```python
from build123d import *

# Parameters (mm, degrees)
F1_DEPTH  = 15
F2_DEPTH  = 15
F3_W      = 7.4589547733
F3_H      = 5.06
F4_DEPTH  = 25
F5_W      = 8.8782840291
F5_H      = 5.06
F6_DEPTH  = 25
F7_W      = 4.8981418308
F7_H      = 5.06
F8_DEPTH  = 25
F9_DEPTH  = 25
F10_DEPTH = 25
F11_R     = 2.5
F12_DEPTH = 25
F14_DEPTH = 15
F11_R_2   = 2
F15_DEPTH = 25


with BuildPart() as f1:
    # F0 (on Top) → F1 (new body)
    with BuildSketch(Plane.XY):
        with BuildLine():
            ThreePointArc((0, -3.5), (2.4748737342, -2.4748737342), (3.5, 0))
            ThreePointArc((3.5, 0), (0, 3.5), (-3.5, 0))
            ThreePointArc((-3.5, 0), (-2.4748737342, -2.4748737342), (0, -3.5))
        make_face()
    extrude(amount=F1_DEPTH)

    # F0 (on Top) → F2 (join)
    with BuildSketch(Plane.XY):
        with BuildLine():
            ThreePointArc((0, -3.5), (2.4748737342, -2.4748737342), (3.5, 0))
            ThreePointArc((3.5, 0), (0, 3.5), (-3.5, 0))
            ThreePointArc((-3.5, 0), (-2.4748737342, -2.4748737342), (0, -3.5))
        make_face()
        with BuildLine():
            ThreePointArc((0, -3.5), (-2.4748737342, -2.4748737342), (-3.5, 0))
            Line((-3.5, 0), (-108.4601820875, -107.1604412839))
            Line((-108.4601820875, -107.1604412839), (-104.9242736666, -110.6956006351))
            Line((-104.9242736666, -110.6956006351), (-37.3017297765, -41.6092114188))
            Line((-37.3017297765, -41.6092114188), (-33.8042539876, -38.0360247309))
            Line((-33.8042539876, -38.0360247309), (-24.8042539876, -28.8411990533))
            Line((-24.8042539876, -28.8411990533), (-21.3067781987, -25.2680123655))
            Line((-21.3067781987, -25.2680123655), (-12.3067781987, -16.0731866878))
            Line((-12.3067781987, -16.0731866878), (-8.8093024098, -12.5))
            Line((-8.8093024098, -12.5), (0, -3.5))
        make_face()
        with BuildLine():
            ThreePointArc((-12.3067781987, -16.0731866878), (-7.2290363366, -17.5450603078), (-8.8093024098, -12.5))
            Line((-8.8093024098, -12.5), (-12.3067781987, -16.0731866878))
        make_face()
        with BuildLine():
            Line((-33.8042539876, -38.0360247309), (-37.3017297765, -41.6092114188))
            ThreePointArc((-37.3017297765, -41.6092114188), (-32.2239879144, -43.0810850387), (-33.8042539876, -38.0360247309))
        make_face()
        with BuildLine():
            ThreePointArc((-24.8042539876, -28.8411990533), (-19.7265121255, -30.3130726732), (-21.3067781987, -25.2680123655))
            Line((-21.3067781987, -25.2680123655), (-24.8042539876, -28.8411990533))
        make_face()
    extrude(amount=F2_DEPTH)

    # F3 (on face) → F4 (join)
    with BuildSketch(Plane(origin=(-1.7863004718, 1.7496234668, 0), x_dir=(-0.6997345473, -0.7144029419, 0), z_dir=(-0.7144029419, 0.6997345473, 0))):
        with Locations((6.178548302, 7.5)):
            Rectangle(F3_W, F3_H)
    extrude(amount=F4_DEPTH)

    # F5 (on face) → F6 (cut)
    with BuildSketch(Plane(origin=(-1.7136995282, -1.7496234668, 0), x_dir=(-0.7144029419, 0.6997345473, 0), z_dir=(0.6997345473, 0.7144029419, 0))):
        with Locations((6.9395523112, 7.5)):
            Rectangle(F5_W, F5_H)
    extrude(amount=F6_DEPTH, mode=Mode.SUBTRACT)

    # F7 (on face) → F8 (cut)
    with BuildSketch(Plane(origin=(-1.7863004718, 1.7496234668, 0), x_dir=(-0.6997345473, -0.7144029419, 0), z_dir=(-0.7144029419, 0.6997345473, 0))):
        with Locations((0, 7.5)):
            Rectangle(F7_W, F7_H)
    extrude(amount=-F8_DEPTH, mode=Mode.SUBTRACT)

    # F9 (cut): a face of the model
    f9_faces = [f1.faces().sort_by_distance(p)[0] for p in [
        (1.7136995282, 1.7496234668, 7.5),
    ]]
    extrude(f9_faces, amount=-F9_DEPTH, mode=Mode.SUBTRACT)

    # F10 (cut): a face of the model
    f10_faces = [f1.faces().sort_by_distance(p)[0] for p in [
        (-23.9697177179, 14.8290140645, 7.5),
    ]]
    extrude(f10_faces, amount=-F10_DEPTH, mode=Mode.SUBTRACT)

    # F11 (on face) → F12 (cut)
    with BuildSketch(Plane(origin=(0, 0, 0), x_dir=(1, 0, 0), z_dir=(0, 0, -1))):
        Circle(F11_R)
    extrude(amount=-F12_DEPTH, mode=Mode.SUBTRACT)

    # F13 (on face) → F14 (join)
    with BuildSketch(Plane.XY.offset(15)):
        with BuildLine():
            Line((-89.8873776378, -95.3331964442), (-104.8883679048, -110.6589176106))
            Line((-104.8883679048, -110.6589176106), (-97.7441379591, -117.6564594926))
            ThreePointArc((-97.7441379591, -117.6564594926), (-95.7182525009, -105.8252374674), (-89.8873776378, -95.3331964442))
        make_face()
        with BuildLine():
            Line((-62.7933306081, -81.9729853935), (-69.9495157778, -74.9637337568))
            Line((-69.9495157778, -74.9637337568), (-84.9671665368, -90.3064760697))
            ThreePointArc((-84.9671665368, -90.3064760697), (-74.5911866059, -84.2480596514), (-62.7933306081, -81.9729853935))
        make_face()
    extrude(amount=-F14_DEPTH)

    # F11 (on face) → F15 (cut)
    with BuildSketch(Plane(origin=(0, 0, 0), x_dir=(1, 0, 0), z_dir=(0, 0, -1))):
        Circle(F11_R)
        with Locations((-34.3678999271, 40.9825995654)):
            Circle(F11_R_2)
        with Locations((-21.8704241382, 28.2145871999)):
            Circle(F11_R_2)
        with Locations((-9.3729483493, 15.4465748344)):
            Circle(F11_R_2)
    extrude(amount=-F15_DEPTH, mode=Mode.SUBTRACT)


solid = f1.part
```
Geometry check sheet. Reference: the model listing, model coordinates, mm. A direction names the side the tool comes from. Coordinates: 2 decimals unless noted, no trailing zeros. Write each loop counter-clockwise with the first axis right and the second up, starting at its lowest first coordinate (ties: lowest second). Pieces come first, ordered by that corner, then holes. Notation, with made-up numbers: M 54.5,69 L 97.5,69 A36 ccw 97.5,106 Z; hole C -32,87.25 d6. An arc over 180 degrees is marked long. One line per item, written item: value. Start each with the question number.
(1) Release check for a two-part mould opening along X. For faces 4 (the face through (-16.87, -20.735, 7.395)), 5 (the face through (-74.75, -84.31, 7.6)), 6 (the face through (-101.366, -114.109, 7.605)), 7 (the face through (-53, -57, 15)) record: released by +X, released by -X, zero draft, split by the parting line, or undercut.
(2) Sectioned sample at A-A, the plane z = 7.25. Enter the section's corners in (x, y).
(3) Tool access check on faces 1 (the face through (-29.367, -33.503, 7.395)), 2 (the face through (2, 2, 4.97)), 3 (the face through (-66.32, -78.52, 7.6)). Record the directions out of +Z, -Z, +X, -X, +Y, -Y that give a thin tool (end or side, any length) a straight path to the whole face; none if there is none.
(4) Scan lines: line 1 along X through (y, z) = (0, 11.5); line 2 along Y through (x, z) = (-8, 6); line 3 along Y through (x, z) = (-65, 1.25). Record each from-to range of solid material in increasing order. Write a range as [from, to].
(5) Sectioned sample at C-C, the plane x = -29.5. Enter the section's corners in (y, z), and give its area (3 significant figures).
(6) Sectioned sample at B-B, the plane y = -53. Enter the section's corners in (x, z), and give its area (3 significant figures).
(7) Depth check by flat-ended pin: pin 1 (4 mm diameter, centred on x = -76, y = -89, fed in from +Z); pin 2 (3 mm diameter, centred on x = -58, z = 7, fed in from +Y); pin 3 (2 mm diameter, centred on x = -44.5, z = 5, fed in from -Y); pin 4 (3 mm diameter, centred on y = -70, z = 5.5, fed in from +X). Enter the tip coordinate at first touch or a pass-through.
Filled sheet:
1. face 4: undercut
1. face 5: released by +X
1. face 6: released by -X
1. face 7: zero draft
2. outline: M -108.46,-107.16 L -104.92,-110.7 L -104.89,-110.66 L -97.74,-117.66 A35.72 cw -89.89,-95.33 L -84.97,-90.31 A35.72 cw -62.79,-81.97 L -69.95,-74.96 L -37.3,-41.61 A3 ccw long -33.8,-38.04 L -24.8,-28.84 A3 ccw long -21.31,-25.27 L -12.31,-16.07 A3 ccw long -8.81,-12.5 L 0,-3.5 A3.5 ccw 0.07,-3.5 L -1.36,-2.1 A2.5 cw -2.07,-1.4 L -3.5,0 Z; hole C -34.37,-40.98 d4; hole C -21.87,-28.21 d4; hole C -9.37,-15.45 d4
3. face 1: +Z, -Z
3. face 2: +X, +Y
3. face 3: +Z, -Z, +X
4. line 1: [-3.5, -2.5], [2.5, 3.5]
4. line 2: [-18.11, -16.9], [-13.99, -12.78], [-11.67, -4.59]
4. line 3: [-82.09, -79.81], [-69.91, -62.79]
5. outline: M -33.64,0 L -26.55,0 L -26.55,15 L -33.64,15 Z
5. area: 106 mm²
6. outline: M -55.41,0 L -48.45,0 L -48.45,15 L -55.41,15 Z
6. area: 104 mm²
7. pin 1: through
7. pin 2: y = -54.11
7. pin 3: y = -49.98
7. pin 4: x = -63.62
